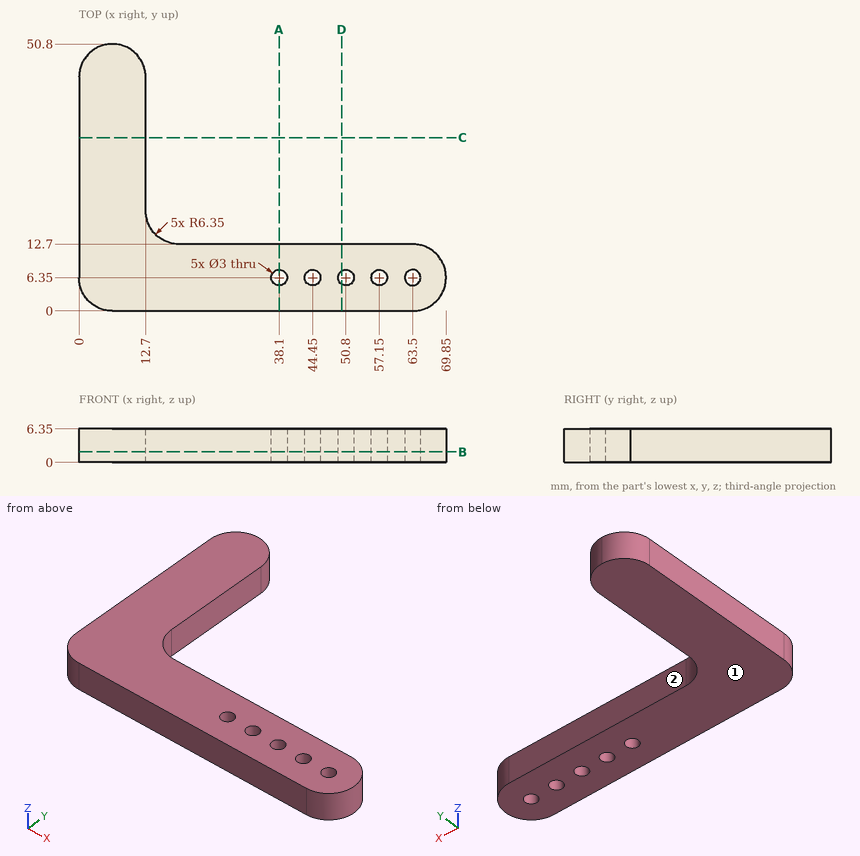
Design review of the part shown in the three views and the two pictorial views. Dimensions are in mm from the part's minimum x, y and z. A direction names the side the tool comes from. Coordinates: 2 decimals unless noted, no trailing zeros. Order: outer loops, then holes, each group sorted by start corner. A loop starts at its lowest first (then second) coordinate and runs counter-clockwise, first axis right, second up.
Item 1: For the marked faces 1 and 2, list the 3-axis set-ups (+Z, -Z, +X, -X, +Y, -Y) from which the entire face can be reached by the end or side of a thin tool; tool diameter is ignored.
Item 2: Take a section at C-C, the plane y = 33. Write out the cut boundary in (x, z).
Item 3: Take a section at A-A, the plane x = 38.1. Write out the cut boundary in (y, z), then the cut area to 3 significant figures.
Item 4: Take a section at D-D, the plane x = 50. Write out the cut boundary in (y, z), then the cut area to 3 significant figures.
Item 5: For line 1 (Y direction, x = 50.8, z = 3.25); line 2 (X direction, y = 38.5, z = 4.25); line 3 (Y direction, x = 39, z = 6), list the stretches that pass through material, from the lowest coordinate up.
Item 6: Take a section at B-B, the plane z = 2. Count the separate pieces of the cut face and the enclosed holes in it, then the cut area to 3 significant figures.
Item 7: For pin 1 Ø2 at (y, z) = (14, 5) entering from -X; pin 2 Ø3 at (x, z) = (41.5, 4.5) entering from +Y; pin 3 Ø1.9 at (y, z) = (32.5, 2) entering from +X, all flat-tipped, find the tip position at first contact; note any pin that passes through.
The answers:
1. face 1: -Z, +X, -X, +Y, -Y
1. face 2: +Z, -Z, +X, +Y
2. outline: (0, 0) - (12.7, 0) - (12.7, 6.35) - (0, 6.35) - close
3. outline: (0, 0) - (4.85, 0) - (4.85, 6.35) - (0, 6.35) - close; (7.85, 0) - (12.7, 0) - (12.7, 6.35) - (7.85, 6.35) - close
3. area: 61.6 mm2
4. outline: (0, 0) - (5.08, 0) - (5.08, 6.35) - (0, 6.35) - close; (7.62, 0) - (12.7, 0) - (12.7, 6.35) - (7.62, 6.35) - close
4. area: 64.5 mm2
5. line 1: y = 0 to 4.85, 7.85 to 12.7
5. line 2: x = 0 to 12.7
5. line 3: y = 0 to 5.15, 7.55 to 12.7
6. separate pieces: 1
6. enclosed holes: 5
6. area: 1,300 mm2
7. pin 1: stops at x = 0
7. pin 2: stops at y = 12.7
7. pin 3: stops at x = 12.7
